Input: part model. Units: mm. Frame: model coordinates. Face numbers are marked on the shaded views. A direction names the side the tool comes from. Give positions to 0.01 mm unless a question says otherwise; leave off trailing zeros. Order: outer loops, then holes, each group sorted by start corner. A loop starts at its lowest first (then second) coordinate and runs counter-clockwise, first axis right, second up. Notation, with made-up numbers: (88, 61) - (127, 61) arc R26 cw to (127, 78) - close; hole circle Ø3 at (44, 7.25). An arc over 180 degrees is marked (long way). Answer in a Markdown table with one row per item. Add a question column.
1. Section query A-A on z = 0. Return loops of the section in (x, y), and give its area (3 significant figures).
2. Mould query, pull axis Y, two halves, no side actions, for the marked faces 3, 4 and 5. Classes: released by +Y, released by -Y, zero draft, split by the parting line, or undercut.
3. Section query C-C on y = 3.25. Return loops of the section in (x, z), and give its area (3 significant figures).
4. Ray query, line 1 (X direction, y = 11, z = 0); line 2 (Y direction, x = 7.25, z = 0.75); line 3 (X direction, y = 7, z = 0). Return the intervals inside material, ascending. Write a range as [from, to].
5. Section query B-B on x = 0. Return loops of the section in (y, z), and give its area (3 significant figures).
6. Section query D-D on y = 9.75. Return loops of the section in (x, z), and give its area (3 significant figures).
7. Access query for the marked faces 1 and 2. Directions: +Z, -Z, +X, -X, +Y, -Y. A direction counts if a zero-diameter tool reaches every point of the face in a straight line with its end or side. Return the directions, or none.
8. Contact query for flat-ended pins moving along their axis: pin 1 (3 mm diameter, centred on y = 1.5, z = -3, fed in from -X); pin 2 (3 mm diameter, centred on x = -4, y = 8.5, fed in from +Z); pin 3 (1.5 mm diameter, centred on x = 3.5, y = 12.5, fed in from -Z). Output: stop coordinate, or through.
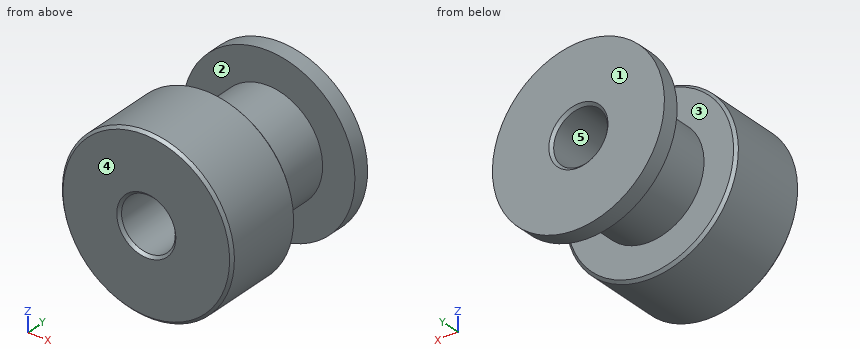
```python
from build123d import *

# Parameters (mm, degrees)
SKETCH1_R           = 8
BOSS_EXTRUDE1_DEPTH = 16
SKETCH2_R           = 2.5
CUT_EXTRUDE1_DEPTH  = 16
SKETCH3_W           = 3
SKETCH3_H           = 7
CHAMFER1_SIZE       = 0.25


with BuildPart() as part:
    # Sketch1 → Boss-Extrude1 (new body)
    with BuildSketch(Plane(origin=(0, 0, 0), x_dir=(1, 0, 0), z_dir=(0, 1, 0))):
        with Locations(Location((0, 0, 0), (0, 0, 270))):
            Circle(SKETCH1_R)
    extrude(amount=BOSS_EXTRUDE1_DEPTH)

    # Sketch2 → Cut-Extrude1 (cut)
    with BuildSketch(Plane(origin=(0, 16, 0), x_dir=(1, 0, 0), z_dir=(0, 1, 0))):
        with Locations(Location((0, 0, 0), (0, 0, 270))):
            Circle(SKETCH2_R)
    extrude(amount=-CUT_EXTRUDE1_DEPTH, mode=Mode.SUBTRACT)

    # Sketch3 → Cut-Revolve1 (revolve, cut)
    with BuildSketch(Plane.XY, mode=Mode.PRIVATE) as cut_revolve1_sk:
        with Locations((6.5, 11)):
            Rectangle(SKETCH3_W, SKETCH3_H)
    revolve(cut_revolve1_sk.sketch.rotate(Axis((0, 16, 0), (0, -1, 0)), 90), axis=Axis((0, 16, 0), (0, -1, 0)), mode=Mode.SUBTRACT)

    # Chamfer1
    chamfer1_edges = [part.edges().sort_by_distance(p)[0] for p in [
        (0, 7.5, -8),
        (0, 0, -8),
        (0, 16, -2.5),
        (0, 0, -2.5),
    ]]
    chamfer(chamfer1_edges, length=CHAMFER1_SIZE)


solid = part.part
```
Answer:
| question | item | result |
|---|---|---|
| 1 | outline | (-8, 0.25) - (-7.75, 0) - (-2.75, 0) - (-2.5, 0.25) - (-2.5, 15.75) - (-2.75, 16) - (-8, 16) - (-8, 14.5) - (-5, 14.5) - (-5, 7.5) - (-7.75, 7.5) - (-8, 7.25) - close; (2.5, 0.25) - (2.75, 0) - (7.75, 0) - (8, 0.25) - (8, 7.25) - (7.75, 7.5) - (5, 7.5) - (5, 14.5) - (8, 14.5) - (8, 16) - (2.75, 16) - (2.5, 15.75) - close |
| 1 | area | 134 mm² |
| 2 | face 3 | undercut |
| 2 | face 4 | released by -Y |
| 2 | face 5 | zero draft |
| 3 | outline | circle Ø16 at (0, 0); hole circle Ø5 at (0, 0) |
| 3 | area | 181 mm² |
| 4 | line 1 | x = [-5, -2.5], [2.5, 5] |
| 4 | line 2 | y = [0, 7.5], [14.5, 16] |
| 4 | line 3 | x = [-8, -2.5], [2.5, 8] |
| 5 | outline | (0, -7.75) - (0.25, -8) - (7.25, -8) - (7.5, -7.75) - (7.5, -5) - (14.5, -5) - (14.5, -8) - (16, -8) - (16, -2.75) - (15.75, -2.5) - (0.25, -2.5) - (0, -2.75) - close; (0, 2.75) - (0.25, 2.5) - (15.75, 2.5) - (16, 2.75) - (16, 8) - (14.5, 8) - (14.5, 5) - (7.5, 5) - (7.5, 7.75) - (7.25, 8) - (0.25, 8) - (0, 7.75) - close |
| 5 | area | 134 mm² |
| 6 | outline | circle Ø10 at (0, 0); hole circle Ø5 at (0, 0) |
| 6 | area | 58.9 mm² |
| 7 | face 1 | +Z, -Z, +X, -X, +Y |
| 7 | face 2 | none |
| 8 | pin 1 | stops at x = -7.86 |
| 8 | pin 2 | stops at z = 7.34 |
| 8 | pin 3 | stops at z = -4.18 |
